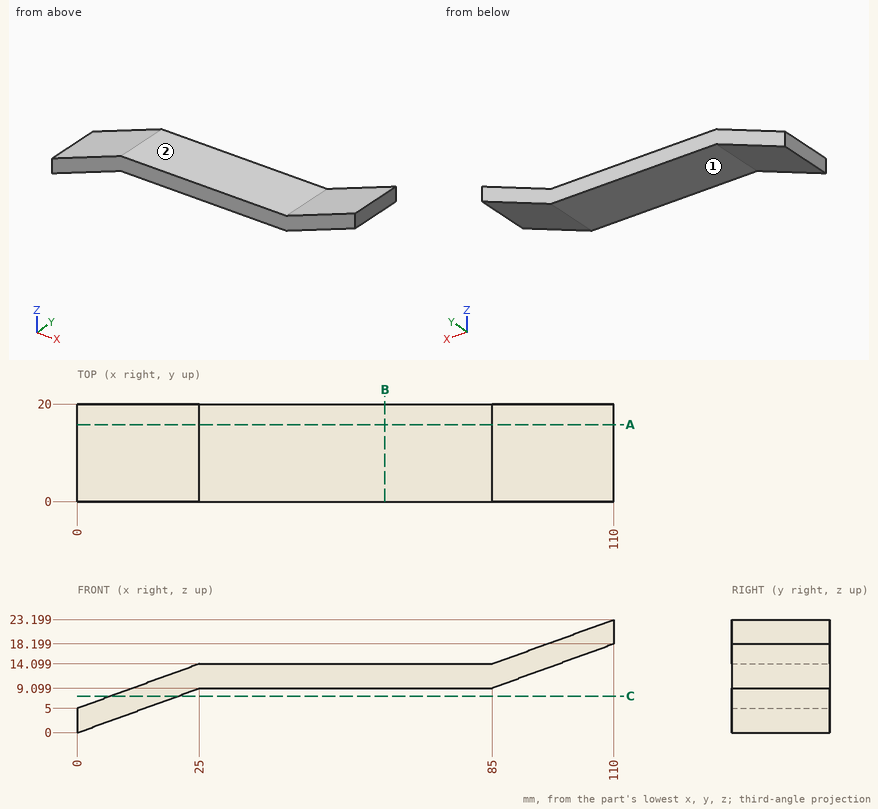
Study the drawing (mm; zero at the part's minimum x, y, z) and answer. A direction names the side the tool comes from. Coordinates: 2 decimals unless noted, no trailing zeros. Write each loop counter-clockwise with the first axis right and the second up, starting at its lowest first coordinate (ties: lowest second). Pieces come first, ordered by that corner, then holes. Notation, with made-up numbers: M -26.75,-16 L 13.25,-16 A28 cw 13.25,15 Z; hole C 25.25,4 d6. An arc over 180 degrees is marked long. Use a Markdown table: item, result. Add a question column.
1. Section A-A (y = 15.75) is taken. Give the vertices of the cut face in (x, z).
2. Straight lines are drawn through the part: line 1 along Z through (x, y) = (37, 14); line 2 along Z through (x, y) = (98, 15.5). For each, find the intervals that lie inside material, in ascending order. Write a range as [from, to].
3. Section B-B (x = 63) is taken. Give the vertices of the cut face in (y, z), plus the area to 3 significant figures.
4. Given P1, Ø12, axis at x = 15, y = 3.5, coming from the -Z side (1 decimal); P2, Ø12, axis at x = 90, y = 18, coming from the -Z side; P3, Ø8, axis at x = 16, y = 16, coming from the -Z side; P4, Ø1, axis at x = 70, z = 7, coming from the +Y side, each flat-ended and moving along its own axis, determine where each tip first touches the part or whether it passes through.
5. Section C-C (z = 7.5) is taken. Give the vertices of the cut face in (x, y), plus the area to 3 significant figures.
6. Which of the six approach directions +Z, -Z, +X, -X, +Y, -Y give full straight-line access (tool end or side, diameter ignored) to the marked faces 1 and 2?
Data:
| question | item | result |
|---|---|---|
| 1 | outline | M 0,0 L 25,9.1 L 85,9.1 L 110,18.2 L 110,23.2 L 85,14.1 L 25,14.1 L 0,5 Z |
| 2 | line 1 | z = [9.1, 14.1] |
| 2 | line 2 | z = [13.83, 18.83] |
| 3 | outline | M 0,9.1 L 20,9.1 L 20,14.1 L 0,14.1 Z |
| 3 | area | 100 mm2 |
| 4 | P1 | stops at z = 3.3 |
| 4 | P2 | stops at z = 9.1 |
| 4 | P3 | stops at z = 4.37 |
| 4 | P4 | passes through |
| 5 | outline | M 6.87,0 L 20.61,0 L 20.61,20 L 6.87,20 Z |
| 5 | area | 275 mm2 |
| 6 | face 1 | -Z, +X, +Y, -Y |
| 6 | face 2 | +Z, -X, +Y, -Y |
